CAD build for the part. Positions are in the model's coordinates, mm. Face numbers are marked on the shaded views. Give positions to 0.01 mm unless a question says otherwise; leave off trailing zeros. Order: outer loops, then holes, each group sorted by start corner. A loop starts at its lowest first (then second) coordinate and runs counter-clockwise, first axis right, second up. Notation, with made-up numbers: (-19, 9) -> (-5, 9) arc R24 cw to (-5, 24) -> close; hole circle Ø5 at (-34, -1). An arc over 180 degrees is marked (long way). Use one line per item in the form item = value. Start each with the question number.
1) Cut at D-D, the plane z = 70. Give the cut face in (x, y), and give its area (3 significant figures).
2) Probe line 1 (X direction, y = 13.5, z = 30); line 2 (Z direction, x = -56, y = 34); line 3 (Y direction, x = 30.5, z = -80). List the from-to ranges inside material, lowest first.
3) Cut at C-C, the plane z = 47. Give the cut face in (x, y).
4) Mould opens along X. For the marked faces 1, 2 and 3 say: pulls with the +X half, pulls with the -X half, needs draft (parallel to the pull), parting line crosses it, or undercut.
5) Cut at B-B, the plane z = -50.8. Give the cut face in (x, y) (3 decimals), and give its area (3 significant figures).
6) Cut at A-A, the plane y = 9.5. Give the cut face in (x, z), and give its area (3 significant figures).
7) Drop flat-ended pins along their axis: P1, Ø4, axis at x = -14.5, y = 24, coming from the -Z side; P2, Ø12.5, axis at y = 23, z = 39, coming from the -X side; P3, Ø4, axis at x = 75.5, z = -67.5, coming from the +Y side; P4, Ø10, axis at x = 0, z = 0, coming from the +Y side. Give the stop position or say it passes through.
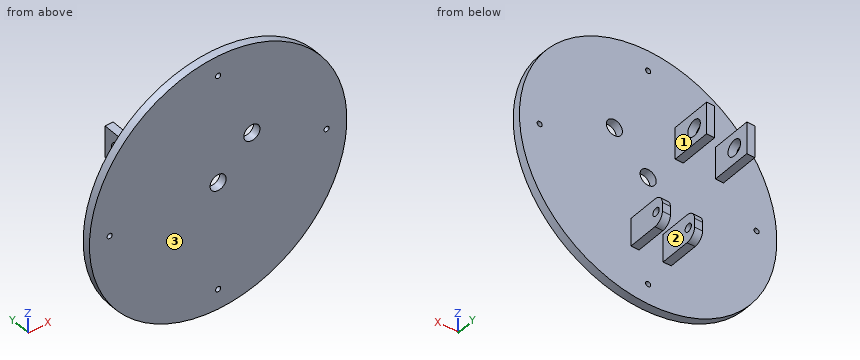
from build123d import *

# Parameters (mm, degrees)
SKETCH1_R                  = 101.6
BOSS_EXTRUDE1_DEPTH        = 6.35
SKETCH2_R                  = 6.35
CUT_EXTRUDE1_DEPTH         = 144.824345992
SKETCH3_W                  = 6.35
SKETCH3_H                  = 25.4
BOSS_EXTRUDE2_DEPTH        = 31.75
CUT_EXTRUDE2_REACH         = 165.994
SKETCH4_R                  = 6.35
SKETCH5_W                  = 6.35
SKETCH5_H                  = 22.225
BOSS_EXTRUDE3_DEPTH        = 31.75
CUT_EXTRUDE3_REACH         = 163.627
SKETCH6_R                  = 3.175
F_10_32_TAPPED_HOLE1_D     = 4.0386
F_10_32_TAPPED_HOLE1_DEPTH = 12.02944
F_10_32_TAPPED_HOLE1_TIP   = 1.213317848
FILLET1_R                  = 7.62
SKETCH9_R                  = 6.35
CUT_EXTRUDE4_DEPTH         = 148.150203873


with BuildPart() as part:
    # Sketch1 → Boss-Extrude1 (new body)
    with BuildSketch(Plane(origin=(0, 0, 0), x_dir=(1, 0, 0), z_dir=(0, 1, 0))):
        with Locations(Location((0, 0, 0), (0, 0, 270))):
            Circle(SKETCH1_R)
    extrude(amount=BOSS_EXTRUDE1_DEPTH)

    # Sketch2 → Cut-Extrude1 (cut, through all)
    with BuildSketch(Plane.XZ):
        with Locations(Location((0, 0, 0), (0, 0, 270))):
            Circle(SKETCH2_R)
    extrude(amount=-CUT_EXTRUDE1_DEPTH, mode=Mode.SUBTRACT)

    # Sketch3 → Boss-Extrude2 (add)
    with BuildSketch(Plane(origin=(0, 6.35, 0), x_dir=(1, 0, 0), z_dir=(0, 1, 0))):
        with Locations((-56.28767, -38.1)):
            Rectangle(SKETCH3_W, SKETCH3_H)
        with Locations((-24.53767, -38.1)):
            Rectangle(SKETCH3_W, SKETCH3_H)
    extrude(amount=BOSS_EXTRUDE2_DEPTH)

    # Cut-Extrude2: up to this face of the body (flat: up to its plane)
    cut_extrude2_end = Plane(part.part.faces().sort_by_distance((-59.46267, 22.225, 38.1))[0])
    # Sketch4 → Cut-Extrude2 (cut, up to the picked face)
    with BuildSketch(Plane(origin=(-21.36267, 0, 0), x_dir=(0, 0, -1), z_dir=(1, 0, 0)), mode=Mode.PRIVATE) as cut_extrude2_sk1:
        with Locations((-38.1, 25.4)):
            Circle(SKETCH4_R)
    cut_extrude2_tool1 = split(extrude(cut_extrude2_sk1.sketch, amount=-CUT_EXTRUDE2_REACH, mode=Mode.PRIVATE), bisect_by=cut_extrude2_end, keep=Keep.BOTH, mode=Mode.PRIVATE)
    add(cut_extrude2_tool1.solids().sort_by(Axis((-21.36267, 25.4, 38.1), (-1, 0, 0)))[0], mode=Mode.SUBTRACT)

    # Sketch5 → Boss-Extrude3 (add)
    with BuildSketch(Plane(origin=(0, 6.35, 0), x_dir=(1, 0, 0), z_dir=(0, 1, 0))):
        with Locations((-15.01267, 50.8)):
            Rectangle(SKETCH5_W, SKETCH5_H)
        with Locations((10.38733, 50.8)):
            Rectangle(SKETCH5_W, SKETCH5_H)
    extrude(amount=BOSS_EXTRUDE3_DEPTH)

    # Cut-Extrude3: up to this face of the body (flat: up to its plane)
    cut_extrude3_end = Plane(part.part.faces().sort_by_distance((13.56233, 22.225, -50.8))[0])
    # Sketch6 → Cut-Extrude3 (cut, up to the picked face)
    with BuildSketch(Plane.ZY.offset(18.18767), mode=Mode.PRIVATE) as cut_extrude3_sk1:
        with Locations((-50.8, 31.75)):
            Circle(SKETCH6_R)
    cut_extrude3_tool1 = split(extrude(cut_extrude3_sk1.sketch, amount=-CUT_EXTRUDE3_REACH, mode=Mode.PRIVATE), bisect_by=cut_extrude3_end, keep=Keep.BOTH, mode=Mode.PRIVATE)
    add(cut_extrude3_tool1.solids().sort_by(Axis((-18.18767, 31.75, -50.8), (1, 0, 0)))[0], mode=Mode.SUBTRACT)

    # #10-32 Tapped Hole1
    with Locations(Plane(origin=(0, 0, 0), x_dir=(-1, 0, 0), z_dir=(0, -1, 0))):
        with Locations((0, 0), (0, -85.599801346), (-85.599801346, 0), (0, 85.599801346), (85.599801346, 0)):
            Hole(F_10_32_TAPPED_HOLE1_D / 2, depth=F_10_32_TAPPED_HOLE1_DEPTH)
            with Locations((0, 0, -(F_10_32_TAPPED_HOLE1_DEPTH + F_10_32_TAPPED_HOLE1_TIP / 2))):  # 118° drill point
                Cone(0, F_10_32_TAPPED_HOLE1_D / 2, F_10_32_TAPPED_HOLE1_TIP, mode=Mode.SUBTRACT)

    # Fillet1
    fillet1_edges = [part.edges().sort_by_distance(p)[0] for p in [
        (-15.01267, 38.1, -39.6875),
        (-15.01267, 38.1, -61.9125),
        (10.38733, 38.1, -39.6875),
        (10.38733, 38.1, -61.9125),
    ]]
    fillet(fillet1_edges, radius=FILLET1_R)

    # Sketch9 → Cut-Extrude4 (cut, through all)
    with BuildSketch(Plane(origin=(0, 6.35, 0), x_dir=(1, 0, 0), z_dir=(0, 1, 0))):
        with Locations(Location((26.662380423, -26.662380423, 0), (0, 0, 270))):
            Circle(SKETCH9_R)
    extrude(amount=-CUT_EXTRUDE4_DEPTH, mode=Mode.SUBTRACT)


solid = part.part
Result:
q1.outline = (-73.64, 0) -> (73.64, 0) -> (73.64, 6.35) -> (-73.64, 6.35) -> close
q1.area = 935 mm²
q2.line_1 = -59.46 to -53.11, -27.71 to -21.36
q2.line_2 = 25.4 to 50.8
q2.line_3 = 0 to 6.35
q3.outline = (-90.08, 0) -> (90.08, 0) -> (90.08, 6.35) -> (-21.36, 6.35) -> (-21.36, 38.1) -> (-27.71, 38.1) -> (-27.71, 6.35) -> (-53.11, 6.35) -> (-53.11, 38.1) -> (-59.46, 38.1) -> (-59.46, 6.35) -> (-90.08, 6.35) -> close
q4.face_1 = pulls with the +X half
q4.face_2 = undercut
q4.face_3 = needs draft
q5.outline = (-87.988, 0) -> (87.988, 0) -> (87.988, 6.35) -> (13.562, 6.35) -> (13.562, 28.575) -> (7.212, 28.575) -> (7.212, 6.35) -> (-11.838, 6.35) -> (-11.838, 28.575) -> (-18.188, 28.575) -> (-18.188, 6.35) -> (-87.988, 6.35) -> close; (-18.188, 34.925) -> (-11.838, 34.925) -> (-11.838, 38.1) -> (-18.188, 38.1) -> close; (7.212, 34.925) -> (13.562, 34.925) -> (13.562, 38.1) -> (7.212, 38.1) -> close
q5.area = 1,440 mm²
q6.outline = (-59.46, 25.4) -> (-53.11, 25.4) -> (-53.11, 50.8) -> (-59.46, 50.8) -> close; (-27.71, 25.4) -> (-21.36, 25.4) -> (-21.36, 50.8) -> (-27.71, 50.8) -> close; (-18.19, -61.91) -> (-11.84, -61.91) -> (-11.84, -39.69) -> (-18.19, -39.69) -> close; (7.21, -61.91) -> (13.56, -61.91) -> (13.56, -39.69) -> (7.21, -39.69) -> close
q6.area = 605 mm²
q7.P1 = -61.91
q7.P2 = -59.46
q7.P3 = 6.35
q7.P4 = through
